```python
from build123d import *

# Parameters (mm, degrees)
BOSS_EXTRUDE1_DEPTH    = 15
BOTTOM_FLANGE_W        = 1312
BOTTOM_FLANGE_H        = 6
BOSS_EXTRUDE2_DEPTH    = 50
F_24_0MM_DOWEL_HOLE1_D = 24
CENTER_HOLE_R          = 25
CUT_EXTRUDE1_DEPTH     = 16


with BuildPart() as part:
    # base plate → Boss-Extrude1 (new body)
    with BuildSketch(Plane.XY):
        with BuildLine():
            Line((0, 0), (1312, 0))
            Line((1312, 0), (1312, 680))
            ThreePointArc((1312, 680), (656, 1336), (0, 680))
            Line((0, 680), (0, 0))
        make_face()
    extrude(amount=BOSS_EXTRUDE1_DEPTH)

    # bottom flange → Boss-Extrude2 (add)
    with BuildSketch(Plane.XY.offset(15)):
        with Locations((656, 3)):
            Rectangle(BOTTOM_FLANGE_W, BOTTOM_FLANGE_H)
    extrude(amount=BOSS_EXTRUDE2_DEPTH)

    # Ø24.0mm Dowel Hole1 (through all)
    with Locations(Plane.XY.offset(15)):
        with Locations((25, 680), (1287, 680), (25, 41), (25, 256), (25, 471), (1287, 41), (1287, 256), (1287, 471), (1238.967985015, 921.473245822), (1102.184378929, 1126.184378929), (897.473245822, 1262.967985015), (656, 1311), (414.526754178, 1262.967985015), (209.815621071, 1126.184378929), (73.032014985, 921.473245822)):
            Hole(F_24_0MM_DOWEL_HOLE1_D / 2)

    # center hole → Cut-Extrude1 (cut, through all)
    with BuildSketch(Plane.XY.offset(15)):
        with Locations((656, 680)):
            Circle(CENTER_HOLE_R)
    extrude(amount=-CUT_EXTRUDE1_DEPTH, mode=Mode.SUBTRACT)


solid = part.part
```
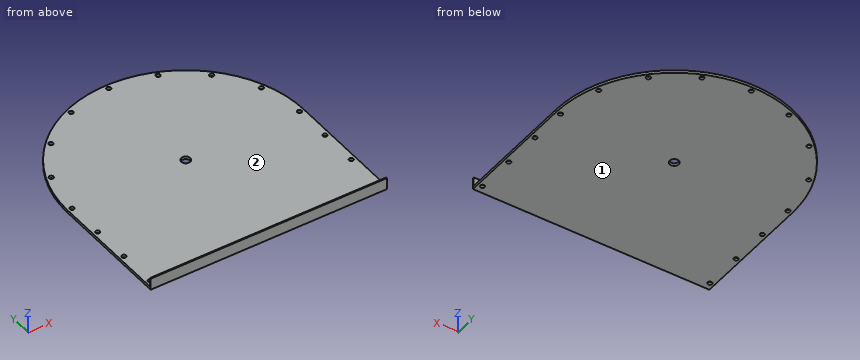
Verification items for the finished model (mm, model axes). Face numbers are marked on the shaded views. A direction names the side the tool comes from. Round coordinates to 2 decimals unless told otherwise and drop trailing zeros. Write each loop counter-clockwise with the first axis right and the second up, starting at its lowest first coordinate (ties: lowest second). Pieces come first, ordered by that corner, then holes.
1. Section check D-D on x = 1026. Enter the section's corners in (y, z).
2. Section check B-B on x = 1203. Enter the section's corners in (y, z), plus the area to 3 significant figures.
3. Scan lines: L1, parallel to Z at x = 596.5, y = 520; L2, parallel to Y at x = 1242.5, z = 16.5; L3, parallel to Y at x = 301.5, z = 10.5. Record each from-to range of solid material in increasing order.
4. Gauge pin test, flat ends, axial feed: P1, Ø5, axis at x = 200.5, z = 58.5, coming from the +Y side; P2, Ø21.5, axis at x = 73.03, y = 921.47, coming from the -Z side; P3, Ø1.5, axis at y = 1162.5, z = 6.5, coming from the +X side. Record the tip position at first contact, or that the pin passes through.
5. Access from +Z, -Z, +X, -X, +Y, -Y to the whole of each face (thin tool, end or side, straight path). Record for the marked faces 1 and 2.
6. Section check A-A on y = 563.5. Enter the section's corners in (x, z).
7. Section check C-C on z = 37.5. Enter the section's corners in (x, y).
Answer:
1. outline: (0, 0) - (1221.7, 0) - (1221.7, 15) - (6, 15) - (6, 65) - (0, 65) - close
2. outline: (0, 0) - (1042.11, 0) - (1042.11, 15) - (6, 15) - (6, 65) - (0, 65) - close
2. area: 15,900 mm2
3. L1: z = 0 to 15
3. L2: y = 0 to 6
3. L3: y = 0 to 1231.97
4. P1: stops at y = 6
4. P2: passes through
4. P3: stops at x = 1101.26
5. face 1: -Z, +X, -X, +Y, -Y
5. face 2: +Z, +X, -X, +Y
6. outline: (0, 0) - (1312, 0) - (1312, 15) - (0, 15) - close
7. outline: (0, 0) - (1312, 0) - (1312, 6) - (0, 6) - close
